Answer from the drawing. Dimensions are ordinates in mm from the lowest x, y and z of the part. Give positions to 0.01 mm unless a question says otherwise; leave off trailing zeros. Loops run counter-clockwise (first coordinate to the right, second up) from the corner with the lowest first, then second, coordinate; pieces in that order, holes last. Notation, with made-up numbers: (67.25, 85.25) -> (84.25, 85.25) arc R26 ccw to (84.25, 111.25) -> close; hole circle Ø9 at (-14.5, 57). An arc over 180 degrees is marked (long way). Write each question's results on one line, items separated by ' | '. Start each with the question number.
Item 1: Section B-B on y = 11 is taken. Write down the section's boundary in (x, z).
Item 2: Find the intervals of material crossed by line 1 (Y direction, x = 569, z = 257.5); line 2 (X direction, y = 4.5, z = 402); line 3 (Z direction, x = 416, y = 57), in increasing order.
Item 3: Each of these flat-tipped pins is pushed along its axis until it touches: P1, Ø12, axis at x = 96.5, y = 66, coming from the +Z side; P2, Ø6, axis at x = 603.5, y = 83, coming from the +Z side; P3, Ø8, axis at y = 72.5, z = 385, coming from the +X side. Where does it stop, or does it pass through?
Item 4: Section C-C on z = 421 is taken. Write down the section's boundary in (x, y).
Item 5: Section A-A on x = 401.5 is taken. Write down the section's boundary in (y, z), and give its area (3 significant figures).
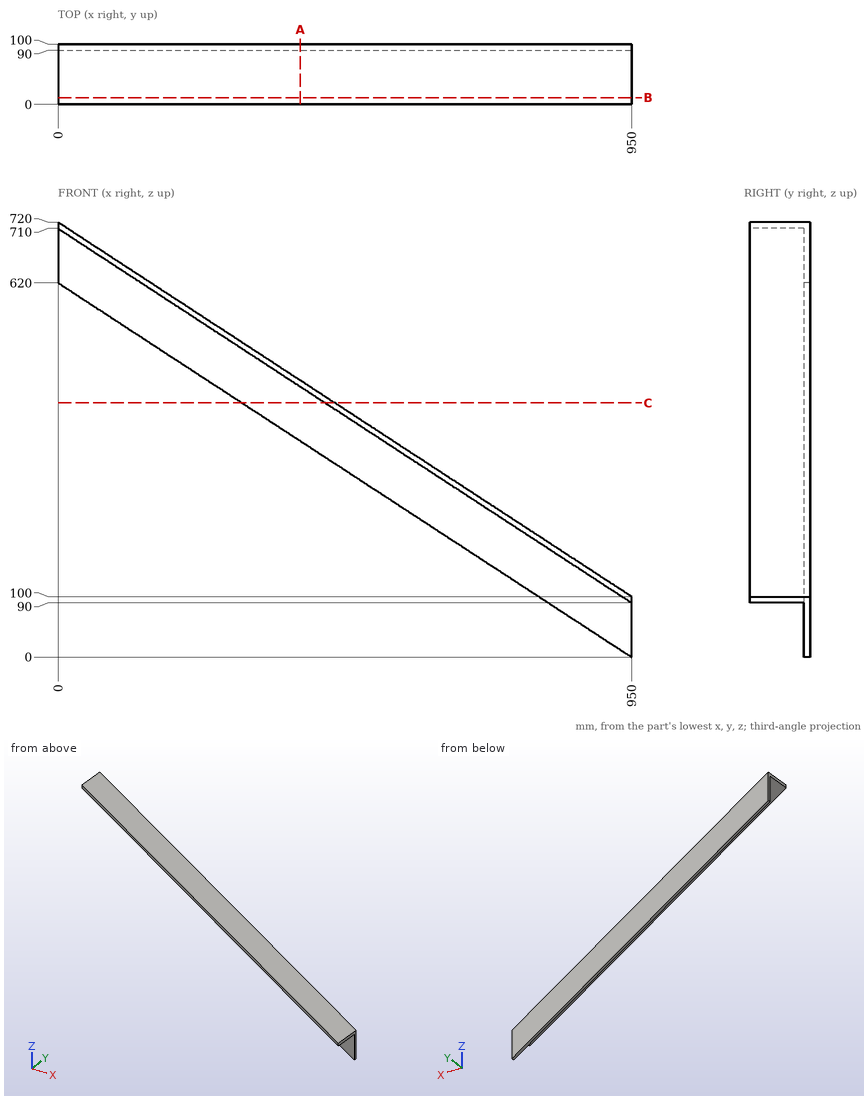
Findings:
1) outline: (0, 710) -> (950, 90) -> (950, 100) -> (0, 720) -> close
2) line 1: 90 to 100 | line 2: 471.94 to 487.26 | line 3: 438.51 to 448.51
3) P1: z = 660.94 | P2: z = 328.09 | P3: x = 519.44
4) outline: (304.92, 90) -> (442.82, 90) -> (442.82, 0) -> (458.15, 0) -> (458.15, 100) -> (304.92, 100) -> close
5) outline: (0, 447.97) -> (90, 447.97) -> (90, 357.97) -> (100, 357.97) -> (100, 457.97) -> (0, 457.97) -> close | area: 1,900 mm2
